Design review of the part shown in the three views and the two pictorial views. Dimensions are in mm from the part's minimum x, y and z. A direction names the side the tool comes from. Give positions to 0.01 mm unless a question says otherwise; leave off trailing zeros. Write each loop counter-clockwise with the first axis right and the second up, starting at its lowest first coordinate (ties: lowest second). Pieces come first, ordered by that corner, then holes.
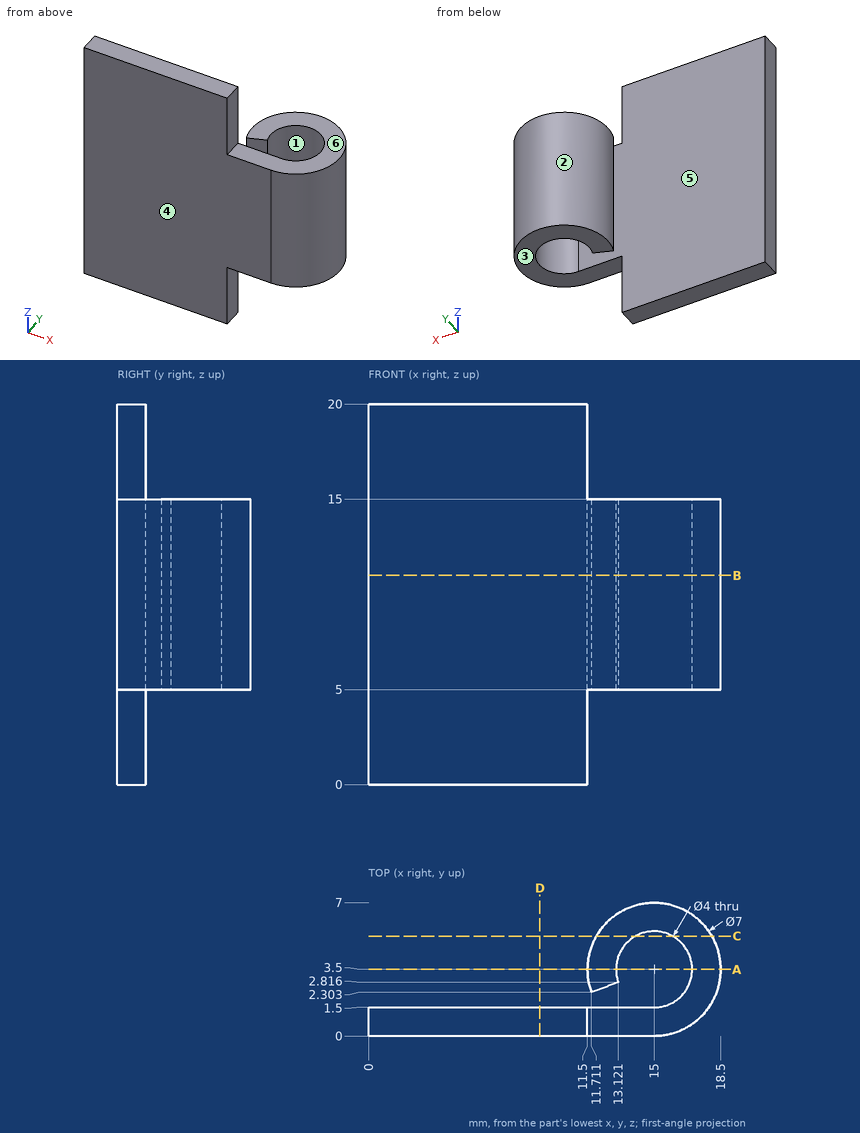
(1) Consider section B-B, the plane z = 11. Give the boundary of the cut face in (x, y).
Resolved:
outline: (0, 0) - (15, 0) arc R3.5 ccw (long way) to (11.71, 2.3) - (13.12, 2.82) arc R2 cw (long way) to (15, 1.5) - (0, 1.5) - close
(2) Consider section D-D, the plane x = 9. Give the boundary of the cut face in (y, z), then the cut area to 3 significant figures.
Resolved:
outline: (0, 0) - (1.5, 0) - (1.5, 20) - (0, 20) - close
area: 30.0 mm2
(3) Consider section A-A, the plane y = 3.5. Give the boundary of the cut face in (x, z).
Resolved:
outline: (11.5, 5) - (13, 5) - (13, 15) - (11.5, 15) - close; (17, 5) - (18.5, 5) - (18.5, 15) - (17, 15) - close
(4) Clearance check with flat-ended pins moving along their axes: P1, Ø2, axis at x = 14, y = 2.5, coming from the -Z side; P2, Ø2, axis at x = 6.5, z = 4.5, coming from the -Y side; P3, Ø4, axis at x = 12.5, z = 11.5, coming from the +Y side; P4, Ø1.5, axis at x = 7.5, y = 3, coming from the +Z side. State where each tip first meets the part, or that it passes through.
Resolved:
P1: stops at z = 5
P2: stops at y = 0
P3: stops at y = 6.96
P4: passes through
(5) Consider section C-C, the plane y = 5.25. Give the boundary of the cut face in (x, z).
Resolved:
outline: (11.97, 5) - (14.03, 5) - (14.03, 15) - (11.97, 15) - close; (15.97, 5) - (18.03, 5) - (18.03, 15) - (15.97, 15) - close
(6) Mouldability with a two-part tool opening along X and no side actions: class the marked faces 1, 2 and 3 as pulls with the +X half, pulls with the -X half, needs draft (parallel to the pull), parting line crosses it, or undercut.
Resolved:
face 1: undercut
face 2: parting line crosses it
face 3: needs draft
(7) To check wall thickness, follow L1, parallel to Y at x = 15, z = 7; L2, parallel to X at y = 3.5, z = 12.75; L3, parallel to Y at x = 9, z = 16.25. State the ranges of each line that lie inside material, in increasing order.
Resolved:
L1: y = 0 to 1.5, 5.5 to 7
L2: x = 11.5 to 13, 17 to 18.5
L3: y = 0 to 1.5
(8) Tool access review of the marked faces 4, 5 and 6: name each direction out of +Z, -Z, +X, -X, +Y, -Y from which nothing blocks a thin tool from reaching the whole face with its end or side.
Resolved:
face 4: +Z, -Z, +X, -X, -Y
face 5: +Z, -Z, -X
face 6: +Z, +X, +Y, -Y
